Verification items for the finished model (mm, model axes). Face numbers are marked on the shaded views. A direction names the side the tool comes from. Round coordinates to 2 decimals unless told otherwise and drop trailing zeros. Write each loop counter-clockwise with the first axis right and the second up, starting at its lowest first coordinate (ties: lowest second). Pieces come first, ordered by that corner, then holes. Notation, with made-up numbers: (-27.5, 15) -> (31.5, 15) arc R15 ccw to (31.5, 33) -> close; hole circle Ø5 at (18, -15.75). An arc over 180 degrees is marked (long way). Use CSV: the item, a comma, the result in double quotes.
```python
from build123d import *

# Parameters (mm, degrees)
EXTRUDE_1_DEPTH     = 20
CUT_EXTRUDE_START   = -3
SKETCH_2_W          = 24
SKETCH_2_H          = 24
CUT_EXTRUDE_1_DEPTH = 14
CUT_EXTRUDE_2_DEPTH = 12
CUT_EXTRUDE_3_DEPTH = 12
SKETCH_5_W          = 6
SKETCH_5_H          = 4
SKETCH_5_W_2        = 4
SKETCH_5_H_2        = 6
CUT_EXTRUDE_4_DEPTH = 30


with BuildPart() as part:
    # 草图1 → 凸台-拉伸1 (new body)
    with BuildSketch(Plane.XY):
        Polygon((0, 28), (0, 0), (28, 0), (28, 6), (24, 6), (6, 24), (6, 28), align=None)
    extrude(amount=EXTRUDE_1_DEPTH)

    # 草图2 → 切除-拉伸1 (cut)
    with BuildSketch(Plane.XY.offset(20).offset(CUT_EXTRUDE_START)):
        with Locations((16, 16)):
            Rectangle(SKETCH_2_W, SKETCH_2_H)
    extrude(amount=-CUT_EXTRUDE_1_DEPTH, mode=Mode.SUBTRACT)

    # 草图3 → 切除-拉伸2 (cut)
    with BuildSketch(Plane(origin=(0, 4, 0), x_dir=(1, 0, 0), z_dir=(0, 1, 0))):
        with BuildLine():
            Line((10, -13), (15, -13))
            ThreePointArc((15, -13), (18, -10), (15, -7))
            Line((15, -7), (10, -7))
            ThreePointArc((10, -7), (7, -10), (10, -13))
        make_face()
    extrude(amount=-CUT_EXTRUDE_2_DEPTH, mode=Mode.SUBTRACT)

    # 草图4 → 切除-拉伸3 (cut)
    with BuildSketch(Plane(origin=(4, 0, 0), x_dir=(0, 0, -1), z_dir=(1, 0, 0))):
        with BuildLine():
            Line((-13, 18), (-13, 13))
            ThreePointArc((-13, 13), (-10, 10), (-7, 13))
            Line((-7, 13), (-7, 18))
            ThreePointArc((-7, 18), (-10, 21), (-13, 18))
        make_face()
    extrude(amount=-CUT_EXTRUDE_3_DEPTH, mode=Mode.SUBTRACT)

    # 草图5 → 切除-拉伸4 (cut)
    with BuildSketch(Plane(origin=(0, 0, 0), x_dir=(-1, 0, 0), z_dir=(0, 0, -1))):
        with Locations((-3, 26)):
            Rectangle(SKETCH_5_W, SKETCH_5_H)
        with Locations((-26, 3)):
            Rectangle(SKETCH_5_W_2, SKETCH_5_H_2)
    extrude(amount=-CUT_EXTRUDE_4_DEPTH, mode=Mode.SUBTRACT)


solid = part.part
```
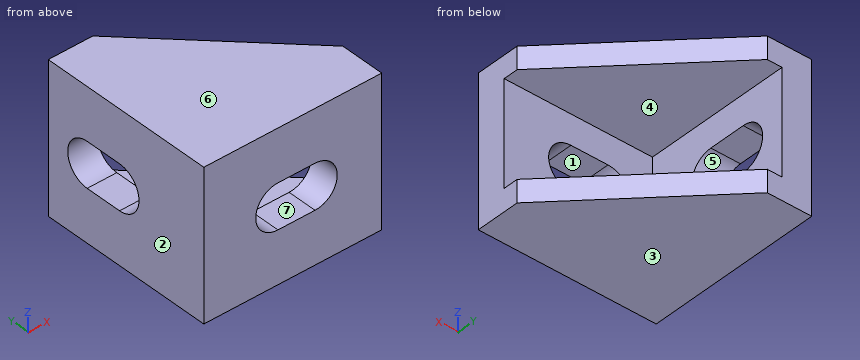
Q1. Material ranges on L1, parallel to Z at x = 5, y = 5.5; L2, parallel to Y at x = 14, z = 3.25, recorded low to high.
Filled in:
L1,"0 to 3, 17 to 20"
L2,"0 to 4"
Q2. Section check D-D (x = 21.75). Record the cut outline in (y, z).
Filled in:
outline,"(0, 0) -> (8.25, 0) -> (8.25, 3) -> (4, 3) -> (4, 17) -> (8.25, 17) -> (8.25, 20) -> (0, 20) -> close"
Q3. Section check B-B (x = 11.75). Record the cut outline in (y, z), plus the area to 4 significant figures.
Filled in:
outline,"(0, 0) -> (18.25, 0) -> (18.25, 3) -> (4, 3) -> (4, 7) -> (0, 7) -> close; (0, 13) -> (4, 13) -> (4, 17) -> (18.25, 17) -> (18.25, 20) -> (0, 20) -> close"
area,"141.5 mm²"
Q4. Section check A-A (y = 14). Record the cut outline in (x, z).
Filled in:
outline,"(0, 0) -> (16, 0) -> (16, 3) -> (4, 3) -> (4, 7) -> (0, 7) -> close; (0, 13) -> (4, 13) -> (4, 17) -> (16, 17) -> (16, 20) -> (0, 20) -> close"
Q5. Access from +Z, -Z, +X, -X, +Y, -Y to the whole of each face (thin tool, end or side, straight path). Record for the marked faces 4, 5, 6 and 7.
Filled in:
face 4,"+X, +Y"
face 5,"+X, -X"
face 6,"+Z, +X, -X, +Y, -Y"
face 7,"+Y, -Y"
Q6. Go/stop test with flat-tipped pins: P1, Ø6, axis at y = 17.5, z = 13.5, coming from the +X side; P2, Ø7, axis at x = 14, z = 8.5, coming from the +Y side; P3, Ø5, axis at x = 19, z = 15, coming from the +Y side; P4, Ø3, axis at x = 21.5, y = 13, coming from the +Z side. Record where each tip stops, or that it passes through.
Filled in:
P1,"x = 4"
P2,"y = 4"
P3,"y = 12.5"
P4,"through"
Q7. Mould release check, pull along Z, two halves, no side actions. Record for the marked faces 1, 2 and 3: released by +Z, released by -Z, zero draft, split by the parting line, or undercut.
Filled in:
face 1,"undercut"
face 2,"zero draft"
face 3,"released by -Z"
Q8. Section check C-C (z = 10). Record the cut outline in (x, y).
Filled in:
outline,"(0, 0) -> (7, 0) -> (7, 4) -> (4, 4) -> (4, 10) -> (0, 10) -> close; (0, 21) -> (4, 21) -> (4, 24) -> (0, 24) -> close; (18, 0) -> (24, 0) -> (24, 4) -> (18, 4) -> close"
